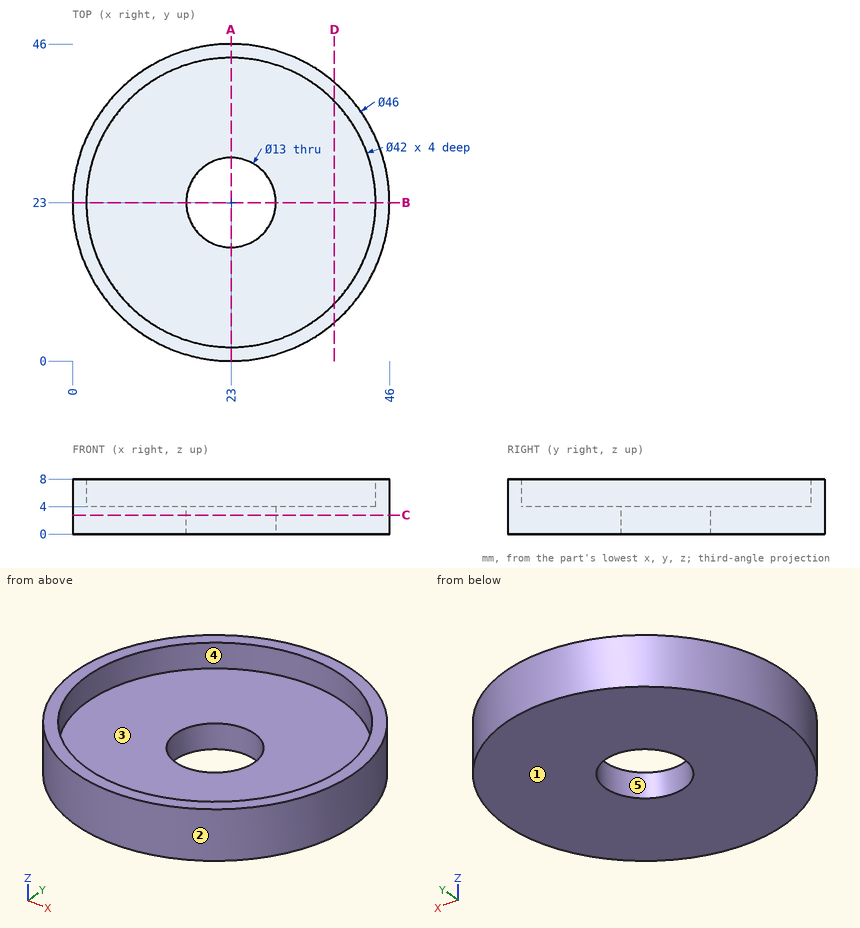
Drawing for the job (mm, zero at the part's lowest x, y, z). A direction names the side the tool comes from. Coordinates: 2 decimals unless noted, no trailing zeros. Loops run counter-clockwise (first coordinate to the right, second up) from the corner with the lowest first, then second, coordinate; pieces in that order, holes last. Notation, with made-up numbers: (36.25, 28.25) - (60.25, 28.25) arc R25 ccw to (60.25, 57.25) - close; hole circle Ø10 at (-28, -19.5). An arc over 180 degrees is marked (long way). Return JSON: item names as keys, results as strings.
1. Drop flat-ended pins along their axis: pin 1 (2 mm diameter, centred on x = 29.5, z = 7, fed in from -Y); pin 2 (1.5 mm diameter, centred on x = 22.5, z = 2, fed in from +Y); pin 3 (12.5 mm diameter, centred on x = 32.5, y = 30, fed in from +Z). Give the stop position or say it passes through.
Result:
{"pin 1": "stops at y = 0.67", "pin 2": "stops at y = 46", "pin 3": "stops at z = 4"}
2. Band-saw the part on D-D (x = 38). Give the cut face in (y, z), and give its area (3 significant figures).
Result:
{"outline": "(5.56, 0) - (40.44, 0) - (40.44, 8) - (37.7, 8) - (37.7, 4) - (8.3, 4) - (8.3, 8) - (5.56, 8) - close", "area": "161 mm2"}
3. Band-saw the part on C-C (z = 2.75). Give the cut face in (x, y), and give its area (3 significant figures).
Result:
{"outline": "circle Ø46 at (23, 23); hole circle Ø13 at (23, 23)", "area": "1,530 mm2"}
4. 3-axis set-ups, long thin cutter, end or side, ignore diameter. For the marked faces 4 and 5: which of +Z, -Z, +X, -X, +Y, -Y reach the whole face in a straight line?
Result:
{"face 4": "+Z", "face 5": "+Z, -Z"}
5. Mould opens along X. For the marked faces 1, 2 and 3 say: released by +X, released by -X, zero draft, split by the parting line, or undercut.
Result:
{"face 1": "zero draft", "face 2": "split by the parting line", "face 3": "undercut"}
6. Band-saw the part on A-A (x = 23). Give the cut face in (y, z).
Result:
{"outline": "(0, 0) - (16.5, 0) - (16.5, 4) - (2, 4) - (2, 8) - (0, 8) - close; (29.5, 0) - (46, 0) - (46, 8) - (44, 8) - (44, 4) - (29.5, 4) - close"}
7. Probe L1, parallel to Y at x = 23, z = 2.2; L2, parallel to Y at x = 23, z = 5.1; L3, parallel to Z at x = 23.5, y = 43. List the from-to ranges inside material, lowest first. Write a range as from..to.
Result:
{"L1": "y = 0..16.5, 29.5..46", "L2": "y = 0..2, 44..46", "L3": "z = 0..4"}
